```python
from build123d import *

# Parameters (mm, degrees)
BOSS_EXTRUDE1_DEPTH = 3
BOSS_EXTRUDE2_DEPTH = 3
CUT_EXTRUDE1_DEPTH  = 4


with BuildPart() as part:
    # Sketch1 → Boss-Extrude1 (new body)
    with BuildSketch(Plane(origin=(0, 0, 0), x_dir=(1, 0, 0), z_dir=(0, 1, 0))):
        Polygon((0, 0), (0, 15), (32.084787993, -1.326860674), (32.084787993, -16.326860674), align=None)
    extrude(amount=BOSS_EXTRUDE1_DEPTH)

    # Sketch2 → Boss-Extrude2 (add)
    with BuildSketch(Plane(origin=(0, 3, 0), x_dir=(1, 0, 0), z_dir=(0, 1, 0))):
        Polygon((25.667830391, -13.061488537), (24.306761694, -15.735988526), (17.889804096, -12.470616391), (19.250872792, -9.796116403), align=None)
        Polygon((12.833915194, -6.530744268), (11.472846497, -9.205244257), (5.055888898, -5.939872122), (6.416957595, -3.265372133), align=None)
    extrude(amount=-BOSS_EXTRUDE2_DEPTH)

    # Sketch3 → Cut-Extrude1 (cut, through all)
    with BuildSketch(Plane(origin=(0, 3, 0), x_dir=(1, 0, 0), z_dir=(0, 1, 0))):
        Polygon((2.673732333, 0.782286134), (2.673732333, 2.925143134), (0, 4.285714857), (0, 2.142857857), align=None)
        Polygon((2.673732333, 5.068000134), (0, 6.428571857), (0, 8.571428857), (2.673732333, 7.210857134), align=None)
        Polygon((2.673732333, 9.353714134), (0, 10.714285857), (0, 12.857142857), (2.673732333, 11.496571134), align=None)
    extrude(amount=-CUT_EXTRUDE1_DEPTH, mode=Mode.SUBTRACT)


solid = part.part
```
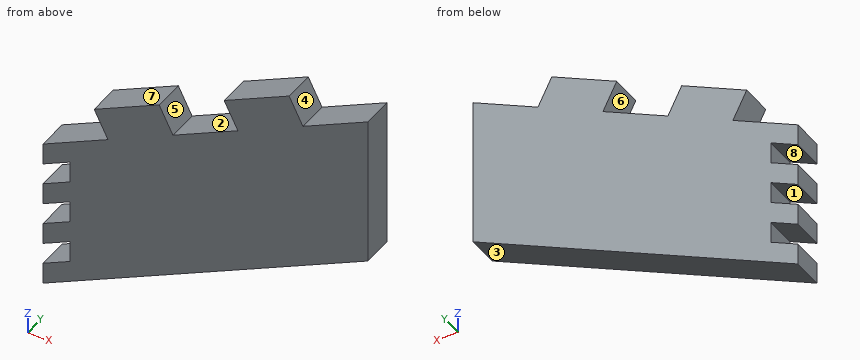
Can you work these out from the model? Positions are in its coordinate system, mm. Face numbers are marked on the shaded views. A direction names the side the tool comes from. Give positions to 0.01 mm unless a question says otherwise; leave off trailing zeros. Loops run counter-clockwise (first coordinate to the right, second up) from the corner with the lowest first, then second, coordinate; pieces in that order, holes last. Notation, with made-up numbers: M -5,34.5 L 43,34.5 A15 cw 43,38.5 Z; hole C 57,25.25 d5. An arc over 180 degrees is marked long. Answer in a Markdown table with one row per item.
1. If I drill on line 1 along Z through (x, y) = (18, 2.35); line 2 along X through (y, z) = (1.2, -5.5); line 3 along Z through (x, y) = (6, 0.65), over which ranges is the centre line in solid material (lowest first)?
Taken from the geometry:
| item | result |
|---|---|
| line 1 | z = -5.84 to 9.16, 12.25 to 12.53 |
| line 2 | x = 0 to 1.82, 2.67 to 18.67 |
| line 3 | z = -11.95 to 3.05, 4.08 to 6.42 |
2. Suppose I cut it at D-D on z = 4. Write out the boundary of the cut face in (x, y), plus the area to 3 significant figures.
Taken from the geometry:
| item | result |
|---|---|
| outline | M 6.04,0 L 32.08,0 L 32.08,3 L 6.04,3 Z |
| area | 78.1 mm² |
3. Suppose I cut it at B-B on y = 2.3. Write out the boundary of the cut face in (x, z), plus the area to 3 significant figures.
Taken from the geometry:
| item | result |
|---|---|
| outline | M 0,-15 L 32.08,1.33 L 32.08,16.33 L 25.67,13.06 L 24.31,15.74 L 17.89,12.47 L 19.25,9.8 L 12.83,6.53 L 11.47,9.21 L 5.06,5.94 L 6.42,3.27 L 0,0 L 0,-2.14 L 2.67,-0.78 L 2.67,-2.93 L 0,-4.29 L 0,-6.43 L 2.67,-5.07 L 2.67,-7.21 L 0,-8.57 L 0,-10.71 L 2.67,-9.35 L 2.67,-11.5 L 0,-12.86 Z |
| area | 507 mm² |
4. For pin 1 Ø1.5 at (x, y) = (19, 0.5) entering from +Z, with a flat end and sliding along its axis, tell me the tip position at first contact or that it passes through.
Taken from the geometry:
| item | result |
|---|---|
| pin 1 | stops at z = 13.42 |
5. Suppose I cut it at C-C on x = 6. Write out the boundary of the cut face in (y, z).
Taken from the geometry:
| item | result |
|---|---|
| outline | M 0,-11.95 L 3,-11.95 L 3,3.05 L 0,3.05 Z; M 0,4.08 L 3,4.08 L 3,6.42 L 0,6.42 Z |
6. Which directions (+Z, -Z, +X, -X, +Y, -Y) give clear straight access to the entire face, cutting with the end or side of a thin tool? Please do the marked faces 5, 6, 7 and 8.
Taken from the geometry:
| item | result |
|---|---|
| face 5 | +Z, +Y, -Y |
| face 6 | -X, +Y, -Y |
| face 7 | +Z, -X, +Y, -Y |
| face 8 | +Y, -Y |
7. Suppose I cut it at A-A on z = 8. Write out the boundary of the cut face in (x, y).
Taken from the geometry:
| item | result |
|---|---|
| outline | M 9.1,0 L 12.09,0 L 12.09,3 L 9.1,3 Z; M 15.72,0 L 32.08,0 L 32.08,3 L 15.72,3 Z |
8. Thinking about a two-plate mould opening in Z: for the marked faces 1, 2, 3 and 4, which applies, released by +Z, released by -Z, zero draft, split by the parting line, or undercut?
Taken from the geometry:
| item | result |
|---|---|
| face 1 | undercut |
| face 2 | undercut |
| face 3 | released by -Z |
| face 4 | released by +Z |
